Geometry: final body of the model. Coordinates: model frame, mm. A direction names the side the tool comes from. Give positions to 0.01 mm unless a question says otherwise; leave off trailing zeros. Order: outer loops, then holes, each group sorted by start corner. A loop starts at its lowest first (then second) coordinate and runs counter-clockwise, first axis right, second up. Notation, with made-up numbers: (8.25, 51.25) -> (55.25, 51.25) arc R19 cw to (55.25, 57.25) -> close; hole circle Ø10 at (-28.75, -18.5). An arc over 180 degrees is marked (long way). Answer in a Markdown table with one row per item. Add a question column.
Q1. Cut plane D-D on x = 268. Return the cut outline in (y, z), and give its area (3 significant figures).
Q2. Set-up query: faces 1 (the face through (255, -17.272, 66)), 2 (the face through (251, -4.064, 75)). Return all of +Z, -Z, +X, -X, +Y, -Y with unobstructed straight access to the full face (end or side cutting, diameter ignored); none if empty.
Q3. Contact query for flat-ended pins moving along their axis: P1, Ø10, axis at x = 238, y = -9, coming from the +Z side; P2, Ø2, axis at x = 244, y = -13, coming from the -Z side; P3, Ø1, axis at y = -14.5, z = 64, coming from the -X side. Output: stop coordinate, or through.
Q4. Pull-direction query (Z, two-part tool) for faces 3 (the face through (269.387, -8.515, 67.315)), 4 (the face through (242.07, -10.76, 75.26)), 5 (the face through (251, 0, 75)); classes: +Z half, -Z half, draft (parallel to the pull), parting line (faces both ways), or undercut.
Q5. Line query: line 1 along Z through (x, y) = (251.5, -5.25); line 2 along X through (y, z) = (-9.5, 74.5); line 3 along Y through (x, z) = (250.5, 74.5). Output: solid intervals per line, ascending. Write a range as from..to.
Q6. Cut plane B-B on y = -11.5. Return the cut outline in (x, z) (3 decimals), and give its area (3 significant figures).
Q7. Cut plane A-A on x = 258.5. Return the cut outline in (y, z), and give its area (3 significant figures).
Q8. Cut plane C-C on z = 83. Return the cut outline in (x, y).
from build123d import *

# Parameters (mm, degrees)
F0_R     = 19.685
F1_DEPTH = 17.272
F2_R     = 9.144
F3_DEPTH = 13.208
F4_R     = 1.999421
F5_DEPTH = 25.4


with BuildPart() as f1:
    # F0 (on Front) → F1 (new body)
    with BuildSketch(Plane.XZ):
        with Locations((251.20312, 74.854024)):
            Circle(F0_R)
    extrude(amount=F1_DEPTH)

    # F2 (on face) → F3 (cut)
    with BuildSketch(Plane.XZ.offset(17.272)):
        with Locations((251.20312, 74.854024)):
            Circle(F2_R)
    extrude(amount=-F3_DEPTH, mode=Mode.SUBTRACT)

    # F4 (on face) → F5 (cut)
    with BuildSketch(Plane.XZ.offset(4.064)):
        with Locations((125.80603, 237.004958)):
            Circle(F4_R)
        with Locations((-78.629516, 256.54611)):
            Circle(F4_R)
        with Locations((-237.004958, 125.80603)):
            Circle(F4_R)
        with Locations((-256.54611, -78.629516)):
            Circle(F4_R)
        with Locations((-125.80603, -237.004958)):
            Circle(F4_R)
        with Locations((78.629516, -256.54611)):
            Circle(F4_R)
        with Locations((237.004958, -125.80603)):
            Circle(F4_R)
    extrude(amount=-F5_DEPTH, mode=Mode.SUBTRACT)


solid = f1.part
Completed:
| question | item | result |
|---|---|---|
| 1 | outline | (-17.27, 64.59) -> (0, 64.59) -> (0, 85.12) -> (-17.27, 85.12) -> close |
| 1 | area | 355 mm² |
| 2 | face 1 | +Z, -Z, +X, -X, -Y |
| 2 | face 2 | -Y |
| 3 | P1 | stops at z = 92.75 |
| 3 | P2 | stops at z = 56.17 |
| 3 | P3 | stops at x = 234.46 |
| 4 | face 3 | parting line |
| 4 | face 4 | undercut |
| 4 | face 5 | draft |
| 5 | line 1 | z = 55.17..65.71, 83.99..94.54 |
| 5 | line 2 | x = 231.52..242.07, 260.34..270.88 |
| 5 | line 3 | y = -4.06..0 |
| 6 | outline | circle Ø39.37 at (251.203, 74.854); hole circle Ø18.288 at (251.203, 74.854) |
| 6 | area | 955 mm² |
| 7 | outline | (-17.27, 56.57) -> (0, 56.57) -> (0, 93.14) -> (-17.27, 93.14) -> (-17.27, 80.36) -> (-4.06, 80.36) -> (-4.06, 69.34) -> (-17.27, 69.34) -> close |
| 7 | area | 486 mm² |
| 8 | outline | (233.28, -17.27) -> (247.05, -17.27) -> (247.05, -4.06) -> (255.36, -4.06) -> (255.36, -17.27) -> (269.12, -17.27) -> (269.12, 0) -> (233.28, 0) -> close |
